The model under review builds one solid part; all positions refer to its coordinate system, in mm. Face numbers are marked on the shaded views. Coordinates: 2 decimals unless noted, no trailing zeros. Write each loop counter-clockwise with the first axis right and the second up, starting at its lowest first coordinate (ties: lowest second). Pieces come first, ordered by that corner, then holes. Notation, with made-up numbers: (89, 83) -> (138, 83) arc R25 cw to (138, 95) -> close; hole circle Ø6 at (2, 18.25). An arc over 180 degrees is marked (long way). Put each result on its own line as item: value. Start each with the question number.
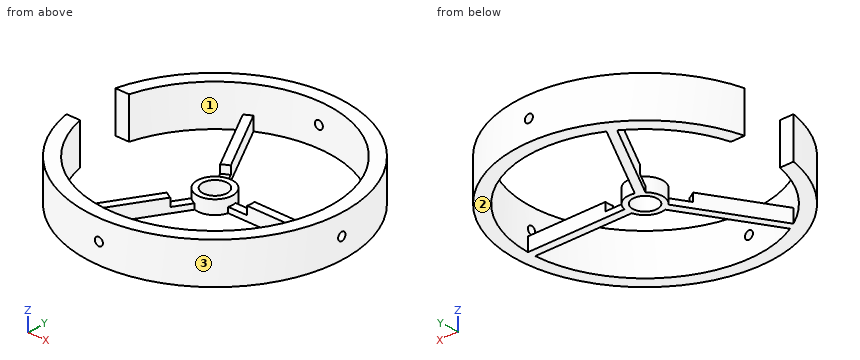
Autodesk Inventor part; units mm, degrees
ref_plane "YZ Plane" through (0, 0, 0) normal (1, 0, 0) x (0, 1, 0)
ref_plane "XZ Plane" through (0, 0, 0) normal (0, 1, 0) x (-1, 0, 0)
ref_plane "XY Plane" through (0, 0, 0) normal (0, 0, 1) x (1, 0, 0)
sketch "Sketch1" plane through (0, 0, 0) normal (0, 0, 1) x (1, 0, 0)
  circle A0 centre (0, 0) radius 47.5 construction
  line L0 (-46.4354, 10) -> (-46.4354, -10) construction
  circle A1 centre (0, 0) radius 42.5 construction
  line L1 (-46.4354, 10) -> (-41.3068, 10)
  line L2 (-46.4354, -10) -> (-41.3068, -10)
  arc A2 (-46.4354, -10) -> (-46.4354, 10) centre (0, 0) ccw
  arc A3 (-41.3068, -10) -> (-41.3068, 10) centre (0, 0) ccw
  circle A4 centre (0, 0) radius 4.5
  circle A5 centre (0, 0) radius 6.5
  line L3 (4.2426, 1.5) -> (47.4763, 1.5)
  line L4 (4.2426, -1.5) -> (47.4763, -1.5)
  arc A6 (4.2426, -1.5) -> (4.2426, 1.5) centre (0, 0) ccw
  arc A7 (47.4763, -1.5) -> (47.4763, 1.5) centre (0, 0) ccw
  line L5 (-3.4204, 2.9242) -> (-25.0372, 40.3657)
  line L6 (-0.8223, 4.4242) -> (-22.4391, 41.8657)
  line L7 (-0.8223, -4.4242) -> (-22.4391, -41.8657)
  line L8 (-3.4204, -2.9242) -> (-25.0372, -40.3657)
  arc A8 (-0.8223, 4.4242) -> (-3.4204, 2.9242) centre (0, 0) ccw
  arc A9 (-3.4204, -2.9242) -> (-0.8223, -4.4242) centre (0, 0) ccw
  arc A10 (-22.4391, 41.8657) -> (-25.0372, 40.3657) centre (0, 0) ccw
  arc A11 (-25.0372, -40.3657) -> (-22.4391, -41.8657) centre (0, 0) ccw
  point P0 (-46.4354, 0)
  dimension "d0" = 95
  dimension "d1" = 20
  dimension "d2" = 5
  dimension "d5" = 9
  dimension "d7" = 3
  dimension "d10" = 360
  dimension "d17" = 13
extrude "Extrusion1" add sketch "Sketch1" along normal blind 15 contours A2 L5 A3 L1 | A2 L6 A3 L5 | A2 L3 A3 L6 | L5 A4 L8 A5 | A5 L6 A4 L5 | A2 L4 A3 L3 | A5 L3 A4 L6 | L8 A4 L7 A5 | A2 L7 A3 L4 | A5 L4 A4 L3 | L7 A4 L4 A5 | L8 A2 L2 A3 | A3 L7 A2 L8
extrude "Extrusion2" add sketch "Sketch1" along normal blind 5 contours A2 L6 A3 L5 | A3 L6 A5 L5 | A5 L6 A4 L5 | A2 L4 A3 L3 | A3 L4 A5 L3 | L8 A4 L7 A5 | A5 L7 A3 L8 | A5 L4 A4 L3 | A3 L7 A2 L8
sketch "Sketch3" plane through (0, 0, 15) normal (0, 0, 1) x (1, 0, 0)
  circle A0 centre (0, 0) radius 4.5
  circle A1 centre (0, 0) radius 6.5
  point P0 (0, 0)
extrude "Extrusion3" cut sketch "Sketch3" against normal blind 10
sketch "Sketch4" plane through (0, 0, 5) normal (0, 0, 1) x (1, 0, 0)
  arc A0 (6.3246, 1.5) -> (-1.8632, 6.2272) centre (0, 0) ccw
  line L0 (42.4735, 1.5) -> (6.3246, 1.5)
  circle A1 centre (0, 0) radius 6.5
  circle A2 centre (0, 0) radius 13.5
  point P0 (0, 0)
  dimension "d18" = 27
extrude "Extrusion4" cut sketch "Sketch4" against normal blind 3
sketch "Sketch5" plane through (0, 0, 0) normal (1, 0, 0) x (0, 1, 0)
  line L0 (-10, 0) -> (10, 0)
  line L1 (10, 0) -> (10, 15)
  line L2 (-10, 15) -> (10, 15)
  line L3 (-10, 0) -> (-10, 15)
  circle A0 centre (0, 7.5) radius 1.5
  point P0 (0, 0)
  point P1 (-10, 7.5)
  point P2 (0, 0)
  dimension "d21" = 3
extrude "Extrusion5" cut sketch "Sketch5" along normal through all contours A0
sketch "Sketch6" plane through (0, 0, 0) normal (0, 1, 0) x (-1, 0, 0)
  circle A0 centre (0, 7.5) radius 1.5
  point P0 (0, 0)
  dimension "d24" = 3
  dimension "d25" = 7.5
extrude "Extrusion6" cut sketch "Sketch6" along normal through all both and the other way through all
properties part number "AA051" material "ABS Plastic"
1. Wall thickness on line 1 (Y direction, x = 0, z = 1.3); line 2 (X direction, y = -3, z = 2); line 3 (X direction, y = 11, z = 3): over which ranges is each line inside the solid? List them lowest first. Write a range as from..to.
2. Consider section A-A on y = 0. State the section outline as (x, z) points, then the cut area to 3 significant figures.
3. Consider section B-B on x = 0. State the section outline as (y, z) points.
4. Consider section C-C on z = 7.5. State the section outline as (x, y) points, then the cut area to 3 significant figures.
5. Consider section D-D on x = 36. State the section outline as (y, z) points.
6. The part is to be moulded in two halves that separate along X. For the marked faces 1, 2 and 3, say which applies: released by +X, released by -X, zero draft, split by the parting line, or undercut.
7. Insertion check: P1, Ø2.5, axis at x = 25, z = 2, coming from the +Y side; P2, Ø1.5, axis at x = -20.5, z = 12, coming from the +Y side; P3, Ø8.5, axis at x = -14.5, y = -29.5, coming from the +Z side; P4, Ø5.5, axis at x = 0, y = 0, coming from the +Z side. Each pin has a flat end and moves straight along its axis. Give the tip position at first contact, or say it passes through.
Output values:
1. line 1: y = -47.5..-42.5, -6.5..-4.5, 4.5..6.5, 42.5..47.5
1. line 2: x = -5.77..-3.35, 3.35..5.77, 42.39..47.41
1. line 3: x = -46.21..-41.05, -8.08..-7.83, 41.05..46.21
2. outline: (-6.5, 0) -> (-4.5, 0) -> (-4.5, 5) -> (-6.5, 5) -> close; (4.5, 0) -> (47.5, 0) -> (47.5, 6) -> (42.5, 6) -> (42.5, 5) -> (13.5, 5) -> (13.5, 2) -> (6.5, 2) -> (6.5, 5) -> (4.5, 5) -> close; (42.5, 9) -> (47.5, 9) -> (47.5, 15) -> (42.5, 15) -> close
2. area: 239 mm^2
3. outline: (-47.5, 0) -> (-42.5, 0) -> (-42.5, 6) -> (-47.5, 6) -> close; (-47.5, 9) -> (-42.5, 9) -> (-42.5, 15) -> (-47.5, 15) -> close; (-6.5, 0) -> (-4.5, 0) -> (-4.5, 5) -> (-6.5, 5) -> close; (4.5, 0) -> (6.5, 0) -> (6.5, 5) -> (4.5, 5) -> close; (42.5, 0) -> (47.5, 0) -> (47.5, 6) -> (42.5, 6) -> close; (42.5, 9) -> (47.5, 9) -> (47.5, 15) -> (42.5, 15) -> close
4. outline: (-46.44, -10) arc R47.5 ccw to (-1.5, -47.48) -> (-1.5, -42.47) arc R42.5 cw to (-41.31, -10) -> close; (-46.44, 10) -> (-41.31, 10) arc R42.5 cw to (-1.5, 42.47) -> (-1.5, 47.48) arc R47.5 ccw to start; (1.5, -47.48) arc R47.5 ccw to (47.48, -1.5) -> (42.47, -1.5) arc R42.5 cw to (1.5, -42.47) -> close; (1.5, 42.47) arc R42.5 cw to (42.47, 1.5) -> (47.48, 1.5) arc R47.5 ccw to (1.5, 47.48) -> close
4. area: 1,270 mm^2
5. outline: (-30.99, 0) -> (-22.59, 0) -> (-22.59, 15) -> (-30.99, 15) -> close; (-1.5, 0) -> (1.5, 0) -> (1.5, 5) -> (-1.5, 5) -> close; (22.59, 0) -> (30.99, 0) -> (30.99, 15) -> (22.59, 15) -> close
6. face 1: undercut
6. face 2: zero draft
6. face 3: split by the parting line
7. P1: stops at y = 41.14
7. P2: stops at y = 43.2
7. P3: stops at z = 5
7. P4: passes through
